Check sheet for the drawn part. Datum: minimum x, y, z corner. Units: mm. Round coordinates to 2 decimals unless told otherwise and drop trailing zeros. Loops run counter-clockwise (first coordinate to the right, second up) from the corner with the lowest first, then second, coordinate; pieces in that order, holes last.
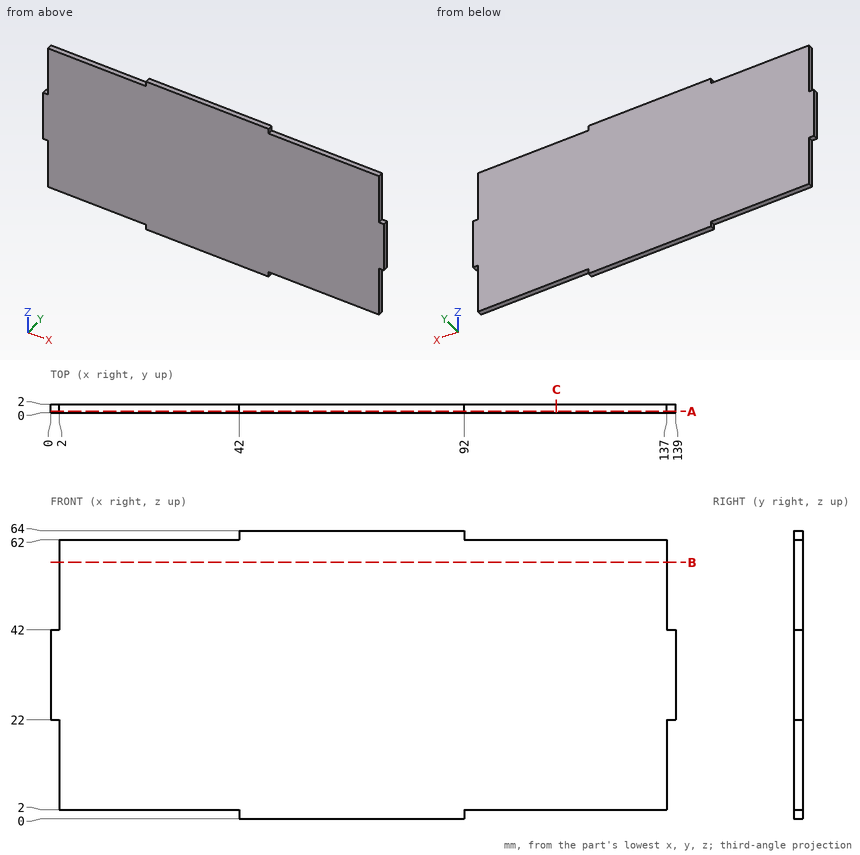
1. Section check C-C (x = 112.5). Enter the section's corners in (y, z).
2. Section check A-A (y = 0.35). Enter the section's corners in (x, z).
3. Gauge pin test, flat ends, axial feed: P1, Ø1, axis at x = 14, y = 1, coming from the -Z side; P2, Ø0.6, axis at y = 1.5, z = 9.5, coming from the -X side; P3, Ø1, axis at y = 1.5, z = 63, coming from the -X side. Record the tip position at first contact, or that the pin passes through.
4. Scan lines: L1, parallel to Z at x = 129, y = 1; L2, parallel to X at y = 0.45, z = 16.5. Record each from-to range of solid material in increasing order.
5. Section check B-B (z = 57). Enter the section's corners in (x, y), then the cut area to 3 significant figures.
Taken from the geometry:
1. outline: (0, 2) - (2, 2) - (2, 62) - (0, 62) - close
2. outline: (0, 22) - (2, 22) - (2, 2) - (42, 2) - (42, 0) - (92, 0) - (92, 2) - (137, 2) - (137, 22) - (139, 22) - (139, 42) - (137, 42) - (137, 62) - (92, 62) - (92, 64) - (42, 64) - (42, 62) - (2, 62) - (2, 42) - (0, 42) - close
3. P1: stops at z = 2
3. P2: stops at x = 2
3. P3: stops at x = 42
4. L1: z = 2 to 62
4. L2: x = 2 to 137
5. outline: (2, 0) - (137, 0) - (137, 2) - (2, 2) - close
5. area: 270 mm2
